from build123d import *

# Parameters (mm, degrees)
BOSS_EXTRUDE1_DEPTH = 70
SKETCH2_R           = 2.2
CUT_EXTRUDE1_DEPTH  = 5.3
FILLET1_R           = 1
SKETCH4_R           = 1.7
CUT_EXTRUDE3_DEPTH  = 10
SKETCH5_R           = 1.75
BOSS_EXTRUDE2_DEPTH = 3
CHAMFER1_SIZE       = 1


with BuildPart() as part:
    # Sketch1 → Boss-Extrude1 (new body)
    with BuildSketch(Plane.XY):
        with BuildLine():
            Line((49, 24), (49, 18.5))
            ThreePointArc((49, 18.5), (49.878679656, 16.378679656), (52, 15.5))
            Line((52, 15.5), (53, 15.5))
            ThreePointArc((53, 15.5), (55.121320344, 14.621320344), (56, 12.5))
            Line((56, 12.5), (56, -12.5))
            ThreePointArc((56, -12.5), (55.121320344, -14.621320344), (53, -15.5))
            Line((53, -15.5), (52, -15.5))
            ThreePointArc((52, -15.5), (49.878679656, -16.378679656), (49, -18.5))
            Line((49, -18.5), (49, -24))
            Line((49, -24), (56, -24))
            ThreePointArc((56, -24), (58.121320344, -23.121320344), (59, -21))
            Line((59, -21), (59, 21))
            ThreePointArc((59, 21), (58.121320344, 23.121320344), (56, 24))
            Line((56, 24), (49, 24))
        make_face()
    extrude(amount=BOSS_EXTRUDE1_DEPTH)

    # Sketch2 → Cut-Extrude1 (cut)
    with BuildSketch(Plane(origin=(0, 0, 0), x_dir=(-1, 0, 0), z_dir=(0, 0, -1))):
        with Locations((-54, -19)):
            Circle(SKETCH2_R)
        with Locations((-54, 19)):
            Circle(SKETCH2_R)
    cut_extrude1 = extrude(amount=-CUT_EXTRUDE1_DEPTH, mode=Mode.SUBTRACT)

    # Mirror1: Cut-Extrude1 across plane
    add(cut_extrude1.mirror(Plane(origin=(0, 0, 35), x_dir=(1, 0, 0), z_dir=(0, 0, -1))), mode=Mode.SUBTRACT)

    # Fillet1
    fillet1_edges = [part.edges().sort_by_distance(p)[0] for p in [
        (49, -24, 35),
    ]]
    fillet(fillet1_edges, radius=FILLET1_R)

    # Sketch4 → Cut-Extrude3 (cut)
    with BuildSketch(Plane(origin=(59, 0, 0), x_dir=(0, 0, -1), z_dir=(1, 0, 0))):
        with Locations(Location((-42, 0, 0), (0, 0, 90))):
            Circle(SKETCH4_R)
        with Locations(Location((-31.5, 6.062177826, 0), (0, 0, 90))):
            Circle(SKETCH4_R)
        with Locations(Location((-31.5, -6.062177826, 0), (0, 0, 90))):
            Circle(SKETCH4_R)
    extrude(amount=-CUT_EXTRUDE3_DEPTH, mode=Mode.SUBTRACT)

    # Sketch5 → Boss-Extrude2 (add)
    with BuildSketch(Plane.XZ.offset(-24)):
        with BuildLine():
            Line((49, 2.5), (42, 2.5))
            ThreePointArc((42, 2.5), (39.878679656, 3.378679656), (39, 5.5))
            Line((39, 5.5), (39, 64.5))
            ThreePointArc((39, 64.5), (39.878679656, 66.621320344), (42, 67.5))
            Line((42, 67.5), (49, 67.5))
            Line((49, 67.5), (49, 2.5))
        make_face()
        with Locations(Location((44, 62.5, 0), (0, 0, 270))):
            Circle(SKETCH5_R, mode=Mode.SUBTRACT)
        with Locations(Location((44, 7.5, 0), (0, 0, 90))):
            Circle(SKETCH5_R, mode=Mode.SUBTRACT)
    extrude(amount=BOSS_EXTRUDE2_DEPTH)

    # Chamfer1
    chamfer1_edges = [part.edges().sort_by_distance(p)[0] for p in [
        (49, 21, 35),
        (49, 22.5, 2.5),
        (49, 22.5, 67.5),
    ]]
    chamfer(chamfer1_edges, length=CHAMFER1_SIZE)


solid = part.part
Read the model definition and answer for the solid it produces. Units are mm, in the model's axes. A direction names the side the tool comes from. Round coordinates to 2 decimals unless told otherwise and drop trailing zeros. Write each loop counter-clockwise with the first axis right and the second up, starting at its lowest first coordinate (ties: lowest second). Pieces come first, ordered by that corner, then holes.
1. Which of the six approach directions +Z, -Z, +X, -X, +Y, -Y give full straight-line access (tool end or side, diameter ignored) to faces 1 (the face through (49, -21, 35)), 2 (the face through (55.14, -14.6, 34.51)), 3 (the face through (55.746, 17.661, 2.613))?
2. The part is cut by section A-A, the plane z = 42. Determine the outline of the cut face in (x, y), then the cut area to 3 significant figures.
3. The part is cut by section C-C, the plane x = 54. Determine the outline of the cut face in (y, z), then the cut area to 3 significant figures.
4. The part is cut by section B-B, the plane y = 0. Determine the outline of the cut face in (x, z), then the cut area to 3 significant figures.
5. Given pin 1 Ø1.3 at (x, y) = (54, -19.5) entering from -Z; pin 2 Ø4.5 at (y, z) = (0, 42) entering from -X; pin 3 Ø3.5 at (y, z) = (-22, 19) entering from -X, each flat-ended and moving along its own axis, determine where each tip first touches the part or whether it passes through.
6. Straight lines are drawn through the part: L1, parallel to Y at x = 54, z = 67.5; L2, parallel to X at y = -20.5, z = 39; L3, parallel to Z at x = 58.25, y = 5.5. For each, find the intervals that lie inside material, in ascending order.
7. Determine the mould class of faces 4 (the face through (58.1, -23.14, 34.51)), 5 (the face through (45, 23, 2.5)), 6 (the face through (54, -19, 64.7)) for opening direction X: pulls with the +X half, pulls with the -X half, needs draft (parallel to the pull), parting line crosses it, or undercut.
8. The part is cut by section D-D, the plane z = 31.5. Determine the outline of the cut face in (x, y).
Values:
1. face 1: +Z, -Z, -X, -Y
1. face 2: +Z, -Z, -X
1. face 3: -Z
2. outline: (39, 21) - (48, 21) - (49, 20) - (49, 18.5) arc R3 ccw to (52, 15.5) - (53, 15.5) arc R3 cw to (56, 12.5) - (56, 1.7) - (59, 1.7) - (59, 21) arc R3 ccw to (56, 24) - (39, 24) - close; (49, -23) arc R1 ccw to (50, -24) - (56, -24) arc R3 ccw to (59, -21) - (59, -1.7) - (56, -1.7) - (56, -12.5) arc R3 cw to (53, -15.5) - (52, -15.5) arc R3 ccw to (49, -18.5) - close
2. area: 279 mm2
3. outline: (-24, 0) - (-21.2, 0) - (-21.2, 5.3) - (-16.8, 5.3) - (-16.8, 0) - (-15.33, 0) - (-15.33, 70) - (-16.8, 70) - (-16.8, 64.7) - (-21.2, 64.7) - (-21.2, 70) - (-24, 70) - close; (15.33, 0) - (16.8, 0) - (16.8, 5.3) - (21.2, 5.3) - (21.2, 0) - (24, 0) - (24, 70) - (21.2, 70) - (21.2, 64.7) - (16.8, 64.7) - (16.8, 70) - (15.33, 70) - close
3. area: 1,120 mm2
4. outline: (56, 0) - (59, 0) - (59, 40.3) - (56, 40.3) - close; (56, 43.7) - (59, 43.7) - (59, 70) - (56, 70) - close
4. area: 200 mm2
5. pin 1: stops at z = 5.3
5. pin 2: stops at x = 56
5. pin 3: stops at x = 49
6. L1: y = -24 to -21.2, -16.8 to -15.33, 15.33 to 16.8, 21.2 to 24
6. L2: x = 49 to 59
6. L3: z = 0 to 29.9, 33.1 to 70
7. face 4: pulls with the +X half
7. face 5: needs draft
7. face 6: undercut
8. outline: (39, 21) - (48, 21) - (49, 20) - (49, 18.5) arc R3 ccw to (52, 15.5) - (53, 15.5) arc R3 cw to (56, 12.5) - (56, 7.76) - (59, 7.76) - (59, 21) arc R3 ccw to (56, 24) - (39, 24) - close; (49, -23) arc R1 ccw to (50, -24) - (56, -24) arc R3 ccw to (59, -21) - (59, -7.76) - (56, -7.76) - (56, -12.5) arc R3 cw to (53, -15.5) - (52, -15.5) arc R3 ccw to (49, -18.5) - close; (56, -4.36) - (59, -4.36) - (59, 4.36) - (56, 4.36) - close
